Here's how the part is built. I have some questions about the finished solid (model axes, mm). A direction names the side the tool comes from. Round coordinates to 2 decimals unless told otherwise and drop trailing zeros. Write each loop counter-clockwise with the first axis right and the second up, starting at its lowest first coordinate (ties: lowest second). Pieces come first, ordered by that corner, then holes. Notation, with made-up numbers: (7, -14) - (56, -14) arc R30 cw to (56, 8) - close; hole circle Ø5 at (21.5, 11). An arc over 180 degrees is marked (long way). One line per question, with ' | ' between items. Start each with the question number.
(1) If I drill on L1, parallel to Y at x = 6.5, z = 16; L2, parallel to Z at x = -37, y = 51.5, over which ranges is the centre line in solid material (lowest first)?
(2) Thinking about a two-plate mould opening in Y: for faces 6 (the flat face through (-46, 50, 14.204)), 7 (the cylindrical face through (-38.9, 57.43, 15.04)), 8 (the flat face through (-34, 57, 15)), which applies, pulls with the +Y half, pulls with the -Y half, needs draft (parallel to the pull), parting line crosses it, or undercut?
(3) Will these pins go through, and if not, where does the flat tip stop? pin 1 (4.5 mm diameter, centred on y = 53.5, z = -14, fed in from -X); pin 2 (0.9 mm diameter, centred on x = -43, z = -15, fed in from +Y); pin 3 (6.5 mm diameter, centred on x = -35.5, y = 54, fed in from +Z).
(4) Imagine slicing it at A-A (z = -5.5). Write out the boundary of the cut face in (x, y).
(5) For faces 1 (the flat face through (-43, 50, 14.922)), 2 (the flat face through (-36, 57.4, -12.5)), 3 (the flat face through (-38.5, 54, -15)), 4 (the flat face through (-35.6, 57.2, -17.5)), 5 (the flat face through (-35.6, 57.2, 17.5)), which set-ups out of +Z, -Z, +X, -X, +Y, -Y let a thin tool reach every point of the face, with its end or its side?
(6) Imagine slicing it at B-B (x = -18). Write out the boundary of the cut face in (y, z), plus the area to 3 significant figures.
from build123d import *

# Parameters (mm, degrees)
SCHIZZO1_W               = 97
SCHIZZO1_H               = 52
ESTRUSIONE1_DEPTH        = 22.5
RACCORDO1_R              = 1
ESTRUSIONE2_DEPTH        = 17.5
SCHIZZO4_W               = 33.983715523
SCHIZZO4_H               = 25
TAGLIO_ESTRUSIONE2_DEPTH = 35
SCHIZZO5_W               = 3.076923077
SCHIZZO5_H               = 0.820512821
TAGLIO_ESTRUSIONE3_DEPTH = 5


with BuildPart() as part:
    # Schizzo1 → Estrusione1 (new, symmetric)
    with BuildSketch(Plane.XY):
        with Locations((0, 26)):
            Rectangle(SCHIZZO1_W, SCHIZZO1_H)
    extrude(amount=ESTRUSIONE1_DEPTH, both=True)

    # Raccordo1
    raccordo1_edges = [part.edges().sort_by_distance(p)[0] for p in [
        (48.5, 26, 22.5),
        (0, 52, 22.5),
        (-48.5, 26, 22.5),
        (0, 52, -22.5),
        (48.5, 26, -22.5),
        (0, 0, -22.5),
        (-48.5, 26, -22.5),
        (0, 0, 22.5),
        (-48.5, 52, 0),
        (48.5, 52, 0),
        (48.5, 0, 0),
        (-48.5, 0, 0),
    ]]
    fillet(raccordo1_edges, radius=RACCORDO1_R)

    # Schizzo3 → Estrusione2 (add, symmetric)
    with BuildSketch(Plane.XY):
        with BuildLine():
            Line((-38.5, 52), (-38.5, 56))
            ThreePointArc((-38.5, 56), (-38.207106781, 56.707106781), (-37.5, 57))
            Line((-37.5, 57), (-29.5, 57))
            Line((-29.5, 57), (-29.5, 58))
            Line((-29.5, 58), (-37.5, 58))
            ThreePointArc((-37.5, 58), (-38.914213562, 57.414213562), (-39.5, 56))
            Line((-39.5, 56), (-39.5, 52))
            Line((-39.5, 52), (-38.5, 52))
        make_face()
    extrude(amount=ESTRUSIONE2_DEPTH, both=True)

    # Schizzo4 → Taglio-Estrusione2 (cut)
    with BuildSketch(Plane(origin=(0, 52, 0), x_dir=(-1, 0, 0), z_dir=(0, 1, 0))):
        with Locations((27.266516562, 0)):
            Rectangle(SCHIZZO4_W, SCHIZZO4_H)
    extrude(amount=TAGLIO_ESTRUSIONE2_DEPTH, mode=Mode.SUBTRACT)

    # Schizzo5 → Taglio-Estrusione3 (cut)
    with BuildSketch(Plane(origin=(0, 52, 0), x_dir=(-1, 0, 0), z_dir=(0, 1, 0))):
        Polygon((43.863317921, 14.922376349), (43.863317921, 17.281350708), (44.581266639, 17.281350708), (44.581266639, 14.922376349), (46.940240998, 14.922376349), (46.940240998, 14.204427631), (44.581266639, 14.204427631), (44.581266639, 11.845453272), (43.863317921, 11.845453272), (43.863317921, 14.204427631), (41.504343562, 14.204427631), (41.504343562, 14.922376349), align=None)
        with Locations((43.183620569, -15.012890571)):
            Rectangle(SCHIZZO5_W, SCHIZZO5_H)
    extrude(amount=-TAGLIO_ESTRUSIONE3_DEPTH, mode=Mode.SUBTRACT)


solid = part.part
Check sheet entries:
1) L1: 0 to 52 | L2: -22.37 to 22.37
2) face 6: needs draft | face 7: pulls with the +Y half | face 8: undercut
3) pin 1: x = -48.47 | pin 2: y = 52 | pin 3: z = 22.5
4) outline: (-48.5, 1) arc R1 ccw to (-47.5, 0) - (47.5, 0) arc R1 ccw to (48.5, 1) - (48.5, 51) arc R1 ccw to (47.5, 52) - (-47.5, 52) arc R1 ccw to (-48.5, 51) - close
5) face 1: +Y | face 2: +X, -X, +Y | face 3: +Z, -Z, +X | face 4: -Z, +X, -X, +Y | face 5: +Z, +X, -X, +Y
6) outline: (0, -21.5) arc R1 ccw to (1, -22.5) - (51, -22.5) arc R1 ccw to (52, -21.5) - (52, 21.5) arc R1 ccw to (51, 22.5) - (1, 22.5) arc R1 ccw to (0, 21.5) - close | area: 2,340 mm^2
